Verification items for the finished model (mm, model axes). Coordinates: 2 decimals unless noted, no trailing zeros. Write each loop counter-clockwise with the first axis right and the second up, starting at its lowest first coordinate (ties: lowest second). Pieces come first, ordered by that corner, then holes. Notation, with made-up numbers: M 27.5,46.25 L 47.5,46.25 A13 cw 47.5,68.25 Z; hole C 83,-3 d3. An arc over 180 degrees is marked long. Answer in a Markdown table with one row per item.
from build123d import *

# Parameters (mm, degrees)
CROQUIS1_R              = 2
CROQUIS1_R_2            = 3.675
CROQUIS1_R_3            = 2.5
CROQUIS1_R_4            = 2.45
CROQUIS1_R_5            = 4
SALIENTE_EXTRUIR1_DEPTH = 3
REDONDEO1_R             = 20
REDONDEO2_R             = 20
REDONDEO3_R             = 5


with BuildPart() as part:
    # Croquis1 → Saliente-Extruir1 (new body)
    with BuildSketch(Plane.XY):
        Polygon((-100, -204.2), (100, -204.2), (100, -94.2), (80, 165.8), (-80, 165.8), (-100, -94.2), align=None)
        with Locations((-23.57, 23.57)):
            Circle(CROQUIS1_R, mode=Mode.SUBTRACT)
        with Locations((23.57, 23.57)):
            Circle(CROQUIS1_R, mode=Mode.SUBTRACT)
        with Locations((-23.57, -23.57)):
            Circle(CROQUIS1_R, mode=Mode.SUBTRACT)
        with Locations((23.57, -23.57)):
            Circle(CROQUIS1_R, mode=Mode.SUBTRACT)
        Circle(CROQUIS1_R_2, mode=Mode.SUBTRACT)
        with Locations((-14, -113.7)):
            Circle(CROQUIS1_R_3, mode=Mode.SUBTRACT)
        with Locations(Location((14, -113.7, 0), (0, 0, 180))):
            Circle(CROQUIS1_R_3, mode=Mode.SUBTRACT)
        with Locations((-45, -98.4)):
            Circle(CROQUIS1_R_4, mode=Mode.SUBTRACT)
        with Locations(Location((45, -98.4, 0), (0, 0, 180))):
            Circle(CROQUIS1_R_4, mode=Mode.SUBTRACT)
        with Locations((-80, -175.5)):
            Circle(CROQUIS1_R_4, mode=Mode.SUBTRACT)
        with Locations(Location((80, -175.5, 0), (0, 0, 180))):
            Circle(CROQUIS1_R_4, mode=Mode.SUBTRACT)
        with Locations((0, -43.7)):
            Circle(CROQUIS1_R_3, mode=Mode.SUBTRACT)
        with Locations((0, -92.7)):
            Circle(CROQUIS1_R_3, mode=Mode.SUBTRACT)
        with Locations((53.25, 136.35)):
            Circle(CROQUIS1_R_5, mode=Mode.SUBTRACT)
        with Locations(Location((53.25, 107.25, 0), (0, 0, 180))):
            Circle(CROQUIS1_R_5, mode=Mode.SUBTRACT)
        with Locations((-53.25, 107.25)):
            Circle(CROQUIS1_R_5, mode=Mode.SUBTRACT)
        with Locations(Location((-53.25, 136.35, 0), (0, 0, 180))):
            Circle(CROQUIS1_R_5, mode=Mode.SUBTRACT)
    extrude(amount=SALIENTE_EXTRUIR1_DEPTH)

    # Redondeo1
    redondeo1_edges = [part.edges().sort_by_distance(p)[0] for p in [
        (100, -204.2, 1.5),
        (-100, -204.2, 1.5),
    ]]
    fillet(redondeo1_edges, radius=REDONDEO1_R)

    # Redondeo2
    # the kernel refuses this fillet: 20 mm, written as the material it takes off along each edge
    with BuildSketch(Plane(origin=(100, -94.2, -1.92024052), x_dir=(0, -1, 0), z_dir=(0, 0, 1))) as redondeo2_piece_1:
        with BuildLine():
            CenterArc((REDONDEO2_R * 0.0384048104053, -REDONDEO2_R), REDONDEO2_R, 90, 4.398705355)
            Line((-REDONDEO2_R * 0.0382916884794, -REDONDEO2_R * 0.00294551449842), (0, 0))
            Line((0, 0), (REDONDEO2_R * 0.0384048104053, 0))
        make_face()
    extrude(amount=6.840481041, mode=Mode.SUBTRACT)
    with BuildSketch(Plane(origin=(-100, -94.2, -1.92024052), x_dir=(0, -1, 0), z_dir=(0, 0, 1))) as redondeo2_piece_2:
        with BuildLine():
            CenterArc((REDONDEO2_R * 0.0384048104053, REDONDEO2_R), REDONDEO2_R, 265.601294645, 4.398705355)
            Line((-REDONDEO2_R * 0.0382916884794, REDONDEO2_R * 0.00294551449842), (0, 0))
            Line((0, 0), (REDONDEO2_R * 0.0384048104053, 0))
        make_face()
    extrude(amount=6.840481041, mode=Mode.SUBTRACT)

    # Redondeo3
    redondeo3_edges = [part.edges().sort_by_distance(p)[0] for p in [
        (80, 165.8, 1.5),
        (-80, 165.8, 1.5),
    ]]
    fillet(redondeo3_edges, radius=REDONDEO3_R)


solid = part.part
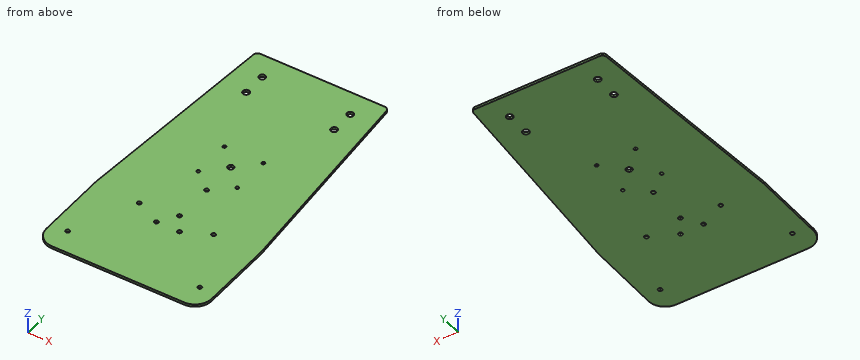
1) Depth check by flat-ended pin: pin 1 (8 mm diameter, centred on x = 80, y = -175.5, fed in from +Z). Enter the tip coordinate at first touch or a pass-through.
Response values:
| item | result |
|---|---|
| pin 1 | stops at z = 3 |
2) Sectioned sample at B-B (x = 53.25). Record the cut outline in (y, z).
Response values:
| item | result |
|---|---|
| outline | M -204.2,0 L 103.25,0 L 103.25,3 L -204.2,3 Z; M 111.25,0 L 132.35,0 L 132.35,3 L 111.25,3 Z; M 140.35,0 L 165.8,0 L 165.8,3 L 140.35,3 Z |
3) Sectioned sample at D-D (y = 107.25). Record the cut outline in (x, z), then the cut area to 3 significant figures.
Response values:
| item | result |
|---|---|
| outline | M -84.5,0 L -57.25,0 L -57.25,3 L -84.5,3 Z; M -49.25,0 L 49.25,0 L 49.25,3 L -49.25,3 Z; M 57.25,0 L 84.5,0 L 84.5,3 L 57.25,3 Z |
| area | 459 mm² |
4) Sectioned sample at C-C (y = 0). Record the cut outline in (x, z) (3 decimals).
Response values:
| item | result |
|---|---|
| outline | M -92.754,0 L -3.675,0 L -3.675,3 L -92.754,3 Z; M 3.675,0 L 92.754,0 L 92.754,3 L 3.675,3 Z |
5) Thickness scan on L1, parallel to Y at x = 53.5, z = 1.75; L2, parallel to Y at x = 14, z = 2.35; L3, parallel to Y at x = 80, z = 1.1. Record the ranges inside material, lowest first. Write a range as [from, to].
Response values:
| item | result |
|---|---|
| L1 | y = [-204.2, 103.26], [111.24, 132.36], [140.34, 165.8] |
| L2 | y = [-204.2, -116.2], [-111.2, 165.8] |
| L3 | y = [-204.2, -177.95], [-173.05, 162.69] |
6) Sectioned sample at A-A (z = 1.5). Give the number of separate pieces and of enclosed holes in the cut face, then the cut area to 3 significant figures.
Response values:
| item | result |
|---|---|
| separate pieces | 1 |
| enclosed holes | 17 |
| area | 68,200 mm² |
